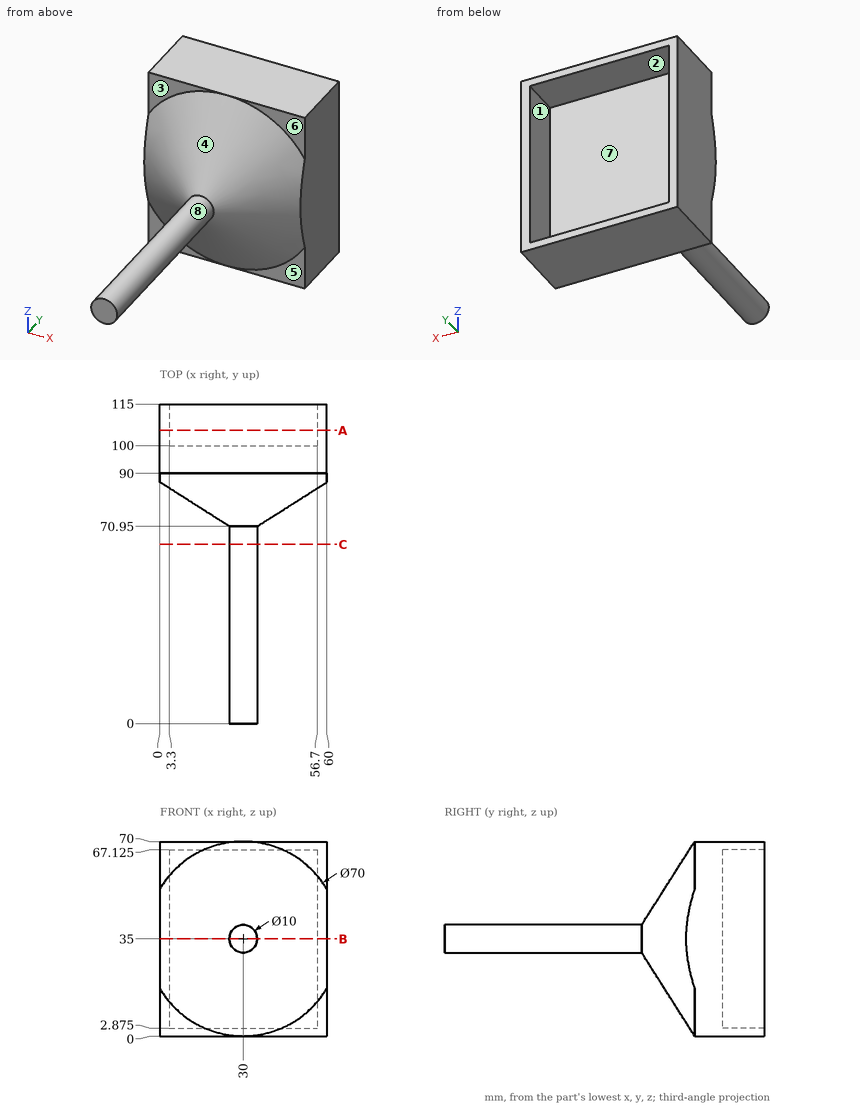
Part print with two shaded views. Sizes in mm from the minimum x, y, z corner. A direction names the side the tool comes from. Round coordinates to 2 decimals unless told otherwise and drop trailing zeros. Loops run counter-clockwise (first coordinate to the right, second up) from the corner with the lowest first, then second, coordinate; pieces in that order, holes last.
Item 1: Saw through at A-A (y = 105.5). List the corners of the cut face in (x, z) (3 decimals), then the cut area to 3 significant figures.
Item 2: Two-plate mould, pull along X, no slides. Class the marked faces 1, 2, 3 and 4: released by +X, released by -X, zero draft, split by the parting line, or undercut.
Item 3: Which spindle directions (+Z, -Z, +X, -X, +Y, -Y) get a long thin tool onto all of the face, cutting with end or side? Do the marked faces 5, 6, 7 and 8. Say none if no direction does.
Item 4: Saw through at C-C (y = 64.5). List the corners of the cut face in (x, z).
Item 5: Drill centre lines: line 1 along Z through (x, y) = (32, 109.5) (3 decimals); line 2 along X through (y, z) = (102.5, 13.5); line 3 along Y through (x, z) = (14, 3). Where is each one in solid material? Low to high.
Item 6: Saw through at B-B (z = 35). List the corners of the cut face in (x, y) (3 decimals), then the cut area to 3 significant figures.
Item 7: Pin check, flat tips, straight feed: P1, Ø6, axis at x = 39, z = 33, coming from the +Y side; P2, Ø8.5, axis at x = 9, z = 4.5, coming from the -Y side; P3, Ø3, axis at x = 14, y = 85.5, coming from the -Z side. Stop position of each tip, or through.
Worked answers:
1. outline: (0, 0) - (60, 0) - (60, 70) - (0, 70) - close; hole (3.3, 2.875) - (56.7, 2.875) - (56.7, 67.125) - (3.3, 67.125) - close
1. area: 769 mm2
2. face 1: undercut
2. face 2: undercut
2. face 3: zero draft
2. face 4: split by the parting line
3. face 5: -Z, +X, -Y
3. face 6: +Z, +X, -Y
3. face 7: +Y
3. face 8: -Y
4. outline: circle Ø10 at (30, 35)
5. line 1: z = 0 to 2.875, 67.125 to 70
5. line 2: x = 0 to 3.3, 56.7 to 60
5. line 3: y = 90 to 100
6. outline: (0, 86.825) - (25, 70.95) - (25, 0) - (35, 0) - (35, 70.95) - (60, 86.825) - (60, 115) - (56.7, 115) - (56.7, 100) - (3.3, 100) - (3.3, 115) - (0, 115) - close
6. area: 2,150 mm2
7. P1: stops at y = 100
7. P2: stops at y = 88.59
7. P3: stops at z = 9.15
